from build123d import *


with BuildPart() as part:
    # Эскиз1 → Повернуть1 (revolve)
    with BuildSketch(Plane.XY, mode=Mode.PRIVATE) as revolve_1_sk:
        Polygon((-2.624106939, 0), (3.925845078, 150), (3.925845078, 0), (10.475797094, 150), (10.475797094, 0), (17.02574911, 150), (15.859832007, 0), (15.311838216, 0), (15.852343113, 110.47254002), (11.684286956, 13.963376462), (10.989801748, -0.846269258), (10.189675666, -0.846269258), (9.467789771, 109.948786309), (4.600142305, 6.147965775), (4.258704841, -1.133064573), (3.526867258, -1.133064573), (3.220264843, 109.948786309), (-1.935686028, 0), align=None)
    revolve(revolve_1_sk.sketch.rotate(Axis((-2.687740891, -0.11397744, 0), (0, 1, 0)), 90), axis=Axis((-2.687740891, -0.11397744, 0), (0, 1, 0)))


solid = part.part
Input: part model. Units: mm. Frame: model coordinates. A direction names the side the tool comes from. Give positions to 0.01 mm unless a question says otherwise; leave off trailing zeros. Order: outer loops, then holes, each group sorted by start corner. A loop starts at its lowest first (then second) coordinate and runs counter-clockwise, first axis right, second up.
Q1. Set-up query: faces 4 (the conical face through (15.98, 73.95, 4.15)), 5 (the flat face through (3.5, -1.133, 1.6)). Return all of +Z, -Z, +X, -X, +Y, -Y with unobstructed straight access to the full face (end or side cutting, diameter ignored); none if empty.
Checked values:
face 4: -Y
face 5: +Z, -Z, +X, -X, -Y
Q2. Section B-B on y = 127. Output: boundary loops of the cut face in (x, z), and give its area (3 significant figures).
Checked values:
outline: circle Ø39.07 at (-2.69, 0); circle Ø26.33 at (-2.69, 0); circle Ø13.23 at (-2.69, 0); hole circle Ø37.42 at (-2.69, 0); hole circle Ø24.32 at (-2.69, 0); hole circle Ø11.22 at (-2.69, 0)
area: 218 mm2
Q3. Ray query, probe 1 along Z at (x, y) = (7, 45.5); probe 2 along X at (y, z) = (135, 7.5); probe 3 along Z at (x, y) = (-13, 112.5). Return the intervals inside material, ascending.
Checked values:
probe 1: z = -16.23 to -15.43, -12.4 to -11.65, -8.91 to -8.02, 8.02 to 8.91, 11.65 to 12.4, 15.43 to 16.23
probe 2: x = -20.79 to -20.21, -13.51 to -12.7, 7.32 to 8.13, 14.83 to 15.42
probe 3: z = -16.46 to -14.85, -8.18 to -5.15, 5.15 to 8.18, 14.85 to 16.46
Q4. Section A-A on y = 18. State how many separate pieces and enclosed holes the cut face has, and give its area (3 significant figures).
Checked values:
separate pieces: 6
enclosed holes: 6
area: 201 mm2
Q5. Contact query for flat-ended pins moving along their axis: pin 1 Ø4 at (y, z) = (17, -0.5) entering from +X; pin 2 Ø4 at (x, y) = (-8, 123.5) entering from +Z; pin 3 Ø4 at (x, y) = (6, 45) entering from -Z. Output: stop coordinate, or through.
Checked values:
pin 1: stops at x = 16.01
pin 2: stops at z = 19.22
pin 3: stops at z = -17.67
Q6. Draft query along Y for faces 1 (the flat face through (9.4, -0.846, -5)), 2 (the conical face through (-8.18, 56.01, -17.43)), 3 (the conical face through (-5.54, 76.05, -1.82)). Return one class per face: +Y half, -Y half, draft (parallel to the pull), parting line (faces both ways), or undercut.
Checked values:
face 1: -Y half
face 2: undercut
face 3: +Y half
